Read the model definition and answer for the solid it produces. Units are mm, in the model's axes. Round coordinates to 2 decimals unless told otherwise and drop trailing zeros. Order: outer loops, then holes, each group sorted by start corner. A loop starts at its lowest first (then second) coordinate and runs counter-clockwise, first axis right, second up. Notation, with made-up numbers: (35, -13) - (85, -13) arc R15 ccw to (85, 6) - close; hole circle Ø1 at (68.5, -10.75). An arc over 180 degrees is marked (long way). Put each result on its own line as item: value. Start each with the question number.
Q1. Find the intervals of material crossed by line 1 along X through (y, z) = (0, -319); line 2 along Z through (x, y) = (31.5, -1.5); line 3 along Y through (x, z) = (1.5, -171), in increasing order. Write a range as from..to.
Q2. Section D-D on x = 10.5 is taken. Give the vertices of the cut face in (y, z), then the cut area to 3 significant figures.
Q3. Section A-A on y = 0 is taken. Give the vertices of the cut face in (x, z), then the cut area to 3 significant figures.
Q4. Each of these flat-tipped pins is pushed along its axis until it touches: pin 1 Ø5 at (x, z) = (1.5, -142) entering from -Y; pin 2 Ø15.5 at (x, z) = (29, -34) entering from +Y; pin 3 Ø8 at (x, z) = (22.5, -46.5) entering from -Y; pin 4 Ø3 at (y, z) = (-9.5, -196) entering from +X. Where does it stop, or does it pass through?
Q5. Section B-B on z = -157.5 is taken. Give the vertices of the cut face in (x, y), then the cut area to 3 significant figures.
Q6. Section C-C on x = -9 is taken. Give the vertices of the cut face in (y, z), then the cut area to 3 significant figures.
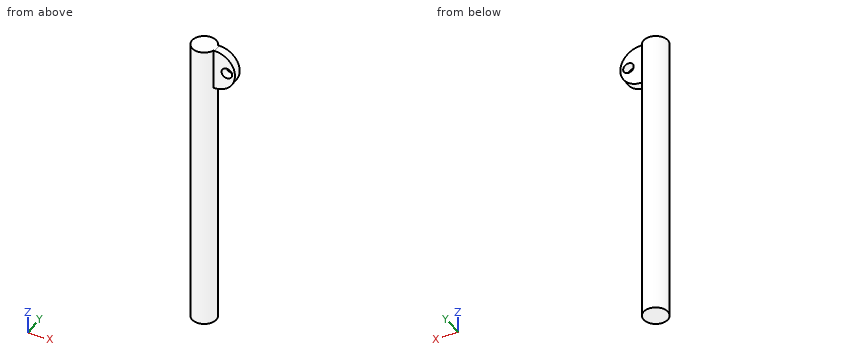
from build123d import *

# Parameters (mm, degrees)
SKETCH1_R                = 17.653
BASE_EXTRUDE_DEPTH       = 431.8
BOSS_EXTRUDE1_DEPTH      = 6.35
BOSS_EXTRUDE1_DEPTH_BACK = 6.35
SKETCH4_R                = 7.62


with BuildPart() as part:
    # Sketch1 → Base-Extrude (new body)
    with BuildSketch(Plane.XY):
        Circle(SKETCH1_R)
    extrude(amount=-BASE_EXTRUDE_DEPTH)

    # Sketch4 → Boss-Extrude1 (add, two sides: drawn at the far end of the back side and taken through both)
    with BuildSketch(Plane(origin=(0, 0, 0), x_dir=(-1, 0, 0), z_dir=(0, 1, 0)).offset(-BOSS_EXTRUDE1_DEPTH_BACK)):
        with BuildLine():
            Line((-9.256612772, -59.074644757), (-9.256612772, 0))
            Line((-9.256612772, 0), (-18.231166151, 0))
            ThreePointArc((-18.231166151, 0), (-47.768488529, -29.537322378), (-18.231166151, -59.074644757))
            Line((-18.231166151, -59.074644757), (-9.256612772, -59.074644757))
        make_face()
        with Locations(Location((-36.011166151, -29.537322378, 0), (0, 0, 90))):
            Circle(SKETCH4_R, mode=Mode.SUBTRACT)
    extrude(amount=BOSS_EXTRUDE1_DEPTH + BOSS_EXTRUDE1_DEPTH_BACK)


solid = part.part
Findings:
1. line 1: -17.65..17.65
1. line 2: -55.93..-35.68, -23.4..-3.15
1. line 3: -17.59..17.59
2. outline: (-14.19, -431.8) - (14.19, -431.8) - (14.19, 0) - (-14.19, 0) - close
2. area: 12,300 mm2
3. outline: (-17.65, -431.8) - (17.65, -431.8) - (17.65, -59.07) - (18.23, -59.07) arc R29.54 ccw to (18.23, 0) - (-17.65, 0) - close; hole circle Ø15.24 at (36.01, -29.54)
3. area: 16,500 mm2
4. pin 1: y = -17.65
4. pin 2: y = 6.35
4. pin 3: y = -6.35
4. pin 4: x = 15.74
5. outline: circle Ø35.31 at (0, 0)
5. area: 979 mm2
6. outline: (-15.19, -431.8) - (15.19, -431.8) - (15.19, 0) - (-15.19, 0) - close
6. area: 13,100 mm2
